Build history of the part. All positions in model axes, mm. Coordinates: 2 decimals unless noted, no trailing zeros. Order: outer loops, then holes, each group sorted by start corner. A loop starts at its lowest first (then second) coordinate and runs counter-clockwise, first axis right, second up. Notation, with made-up numbers: (-21, 23.5) - (-15, 23.5) arc R27 ccw to (-15, 61.5) - close; hole circle Ø8 at (5.5, -8.75). An arc over 180 degrees is marked (long way). Return JSON: item names as keys, results as strings.
from build123d import *

# Parameters (mm, degrees)
F0_W     = 50
F0_H     = 50
F1_DEPTH = 3.2
F2_R     = 5
F3_SIZE  = 1.2


with BuildPart() as f1:
    # F0 (on Top) → F1 (new body)
    with BuildSketch(Plane.XY):
        Rectangle(F0_W, F0_H)
    extrude(amount=F1_DEPTH)

    # F2
    f2_edges = [f1.edges().sort_by_distance(p)[0] for p in [
        (-25, -25, 1.6),
        (25, -25, 1.6),
        (25, 25, 1.6),
        (-25, 25, 1.6),
    ]]
    fillet(f2_edges, radius=F2_R)

    # F3
    f3_edges = [f1.edges().sort_by_distance(p)[0] for p in [
        (0, -25, 0),
        (-23.535534, -23.535534, 0),
        (23.535534, -23.535534, 0),
        (-25, 0, 0),
        (25, 0, 0),
        (-23.535534, 23.535534, 0),
        (23.535534, 23.535534, 0),
        (0, 25, 0),
        (0, -25, 3.2),
        (-23.535534, -23.535534, 3.2),
        (23.535534, -23.535534, 3.2),
        (-25, 0, 3.2),
        (25, 0, 3.2),
        (-23.535534, 23.535534, 3.2),
        (23.535534, 23.535534, 3.2),
        (0, 25, 3.2),
    ]]
    chamfer(f3_edges, length=F3_SIZE)


solid = f1.part
1. Probe L1, parallel to Y at x = -0.5, z = 2.3; L2, parallel to Y at x = 5, z = 2.7; L3, parallel to X at y = 5.5, z = 0.4. List the from-to ranges inside material, lowest first.
Check values:
{"L1": "-24.7 to 24.7", "L2": "-24.3 to 24.3", "L3": "-24.2 to 24.2"}
2. Cut at A-A on z = 2.6. Give the cut face in (x, y).
Check values:
{"outline": "(-24.4, -20) arc R4.4 ccw to (-20, -24.4) - (20, -24.4) arc R4.4 ccw to (24.4, -20) - (24.4, 20) arc R4.4 ccw to (20, 24.4) - (-20, 24.4) arc R4.4 ccw to (-24.4, 20) - close"}
3. Cut at B-B on x = -1.5. Give the cut face in (y, z).
Check values:
{"outline": "(-25, 1.2) - (-23.8, 0) - (23.8, 0) - (25, 1.2) - (25, 2) - (23.8, 3.2) - (-23.8, 3.2) - (-25, 2) - close"}
